from build123d import *

# Parameters (mm, degrees)
F0_W     = 474.98
F0_H     = 266.7
F1_DEPTH = 25.4
F2_W     = 500.38
F2_H     = 292.1
F2_W_2   = 474.98
F2_H_2   = 266.7
F3_DEPTH = 31.75


with BuildPart() as f1:
    # F0 (on Front) → F1 (new body)
    with BuildSketch(Plane.XZ):
        Rectangle(F0_W, F0_H)
    extrude(amount=F1_DEPTH)

    # F2 (on Front) → F3 (join)
    with BuildSketch(Plane.XZ):
        Rectangle(F2_W, F2_H)
        Rectangle(F2_W_2, F2_H_2, mode=Mode.SUBTRACT)
    extrude(amount=F3_DEPTH)


solid = f1.part
Input: part model. Units: mm. Frame: model coordinates. Coordinates: 2 decimals unless noted, no trailing zeros. Order: outer loops, then holes, each group sorted by start corner. A loop starts at its lowest first (then second) coordinate and runs counter-clockwise, first axis right, second up. Notation, with made-up numbers: M 79,52.5 L 83,52.5 A25 ccw 83,84.5 Z; hole C 77,86 d3. An arc over 180 degrees is marked long. Write item = value, one per line. Start each with the question number.
(1) Pull-direction query (Z, two-part tool) for faces 1 (the flat face through (-4, -16, 146.05)), 2 (the flat face through (-3, -25.4, 2)), 3 (the flat face through (-4, 0, 2)); classes: released by +Z, released by -Z, zero draft, split by the parting line, or undercut.
(2) Section B-B on z = -51.5. Output: boundary loops of the cut face in (x, y), and give its area (3 significant figures).
(3) First-contact query: P1, Ø1, axis at x = 168, z = 10.5, coming from the -Y side. Flat tip, straight axial feed; report the tip coordinate or a pass-through.
(4) Line query: line 1 along X through (y, z) = (-29.5, 90.5); line 2 along Z through (x, y) = (-30.5, -26.5); line 3 along Y through (x, z) = (218, -24.5). Output: solid intervals per line, ascending. Write a range as [from, to].
(5) Section A-A on x = 112.5. Output: boundary loops of the cut face in (y, z).
Result set:
q1.face_1 = released by +Z
q1.face_2 = undercut
q1.face_3 = zero draft
q2.outline = M -250.19,-31.75 L -237.49,-31.75 L -237.49,-25.4 L 237.49,-25.4 L 237.49,-31.75 L 250.19,-31.75 L 250.19,0 L -250.19,0 Z
q2.area = 12,900 mm²
q3.P1 = -25.4
q4.line_1 = [-250.19, -237.49], [237.49, 250.19]
q4.line_2 = [-146.05, -133.35], [133.35, 146.05]
q4.line_3 = [-25.4, 0]
q5.outline = M -31.75,-146.05 L 0,-146.05 L 0,146.05 L -31.75,146.05 L -31.75,133.35 L -25.4,133.35 L -25.4,-133.35 L -31.75,-133.35 Z
